```python
from build123d import *

# Parameters (mm, degrees)
SKETCH5_W           = 533.4
SKETCH5_H           = 533.4
SKETCH5_W_2         = 482.6
SKETCH5_H_2         = 482.6
BOSS_EXTRUDE1_DEPTH = 25.4
SKETCH6_W           = 533.4
SKETCH6_H           = 533.4
SKETCH6_W_2         = 482.6
SKETCH6_H_2         = 482.6
BOSS_EXTRUDE2_DEPTH = 25.4


with BuildPart() as part:
    # Sketch2 → Loft1 section 0
    with BuildSketch(Plane.XY.offset(1549.4)):
        with BuildLine():
            Line((-254, -254), (254, -254))
            Line((254, -254), (254, 254))
            Line((254, 254), (-254, 254))
            Line((-254, 254), (-254, -254))
        make_face()
    # Sketch1 → Loft1 section 1
    with BuildSketch(Plane.XY):
        with BuildLine():
            Line((-254, -254), (254, -254))
            Line((254, -254), (254, 254))
            Line((254, 254), (-254, 254))
            Line((-254, 254), (-254, -254))
        make_face()
    loft()

    # Sketch4 → Cut-Loft1 section 0
    with BuildSketch(Plane(origin=(0, 0, 0), x_dir=(-1, 0, 0), z_dir=(0, 0, -1))):
        with BuildLine():
            Line((-241.3, -241.3), (241.3, -241.3))
            Line((241.3, -241.3), (241.3, 241.3))
            Line((241.3, 241.3), (-241.3, 241.3))
            Line((-241.3, 241.3), (-241.3, -241.3))
        make_face()
    # Sketch3 → Cut-Loft1 section 1
    with BuildSketch(Plane.XY.offset(1549.4)):
        with BuildLine():
            Line((241.3, -241.3), (241.3, 241.3))
            Line((241.3, 241.3), (-241.3, 241.3))
            Line((-241.3, 241.3), (-241.3, -241.3))
            Line((-241.3, -241.3), (241.3, -241.3))
        make_face()
    loft(mode=Mode.SUBTRACT)

    # Sketch5 → Boss-Extrude1 (add)
    with BuildSketch(Plane(origin=(0, 0, 0), x_dir=(-1, 0, 0), z_dir=(0, 0, -1))):
        Rectangle(SKETCH5_W, SKETCH5_H)
        Rectangle(SKETCH5_W_2, SKETCH5_H_2, mode=Mode.SUBTRACT)
    extrude(amount=BOSS_EXTRUDE1_DEPTH)

    # Sketch6 → Boss-Extrude2 (add)
    with BuildSketch(Plane.XY.offset(1549.4)):
        Rectangle(SKETCH6_W, SKETCH6_H)
        Rectangle(SKETCH6_W_2, SKETCH6_H_2, mode=Mode.SUBTRACT)
    extrude(amount=BOSS_EXTRUDE2_DEPTH)


solid = part.part
```
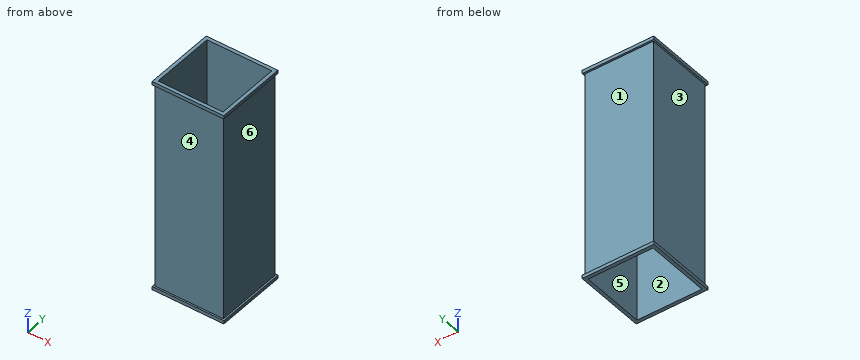
Can you work these out from the model? Positions are in its coordinate system, mm. Face numbers are marked on the shaded views. A direction names the side the tool comes from. Coordinates: 2 decimals unless noted, no trailing zeros. Loops run counter-clockwise (first coordinate to the right, second up) from the corner with the lowest first, then second, coordinate; pieces in that order, holes last. Notation, with made-up numbers: (-15.5, 80) -> (-9.5, 80) arc R25 ccw to (-9.5, 92) -> close; hole circle Ø1 at (36.5, 6.5). An arc over 180 degrees is marked (long way). Answer as a JSON object with one key per item and string values.
1) For the marked faces 4, 5 and 6, which set-ups out of +Z, -Z, +X, -X, +Y, -Y let a thin tool reach every point of the face, with its end or its side?
Results:
{"face 4": "+X, -X, -Y", "face 5": "+Z, -Z", "face 6": "+X, +Y, -Y"}
2) For P1, Ø2, axis at y = 80.5, z = 413.5, coming from the +X side; P2, Ø1, axis at x = -206.5, z = 1410.5, coming from the -Y side; P3, Ø4, axis at x = 80.5, z = 340.5, coming from the +Y side, each with a flat end and sliding along its axis, tell me the tip position at first contact or that it passes through.
Results:
{"P1": "stops at x = 254", "P2": "stops at y = -254", "P3": "stops at y = 254"}
3) If I drill on line 1 (Y direction, x = -206, z = 1082.5); line 2 (Y direction, x = 244.5, z = 213.5), over which ranges is the centre line in solid material (lowest first)?
Results:
{"line 1": "y = -254 to -241.3, 241.3 to 254", "line 2": "y = -254 to 254"}
4) Imagine slicing it at B-B (z = 283.5). Please give me the cut outline in (x, y), then the cut area to 3 significant figures.
Results:
{"outline": "(-254, -254) -> (254, -254) -> (254, 254) -> (-254, 254) -> close; hole (-241.3, -241.3) -> (241.3, -241.3) -> (241.3, 241.3) -> (-241.3, 241.3) -> close", "area": "25,200 mm^2"}
5) Thinking about a two-plate mould opening in X: for the marked faces 1, 2 and 3, which applies, pulls with the +X half, pulls with the -X half, needs draft (parallel to the pull), parting line crosses it, or undercut?
Results:
{"face 1": "needs draft", "face 2": "undercut", "face 3": "pulls with the -X half"}
6) Imagine slicing it at A-A (y = -153). Please give me the cut outline in (x, z).
Results:
{"outline": "(-266.7, -25.4) -> (-241.3, -25.4) -> (-241.3, 1574.8) -> (-266.7, 1574.8) -> (-266.7, 1549.4) -> (-254, 1549.4) -> (-254, 0) -> (-266.7, 0) -> close; (241.3, -25.4) -> (266.7, -25.4) -> (266.7, 0) -> (254, 0) -> (254, 1549.4) -> (266.7, 1549.4) -> (266.7, 1574.8) -> (241.3, 1574.8) -> close"}
